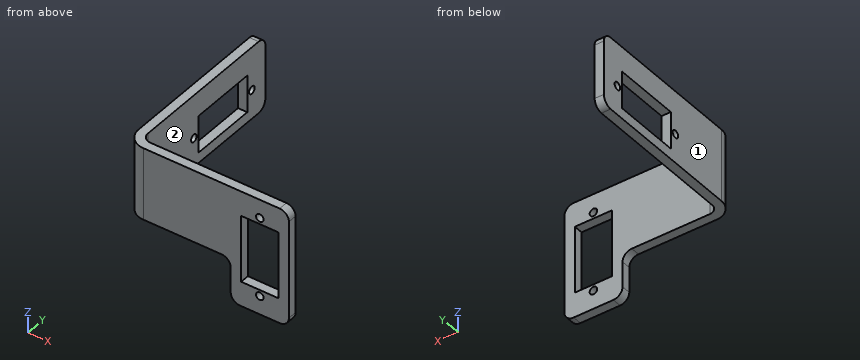
Autodesk Inventor part; units mm, degrees
ref_plane "YZ Plane" through (0, 0, 0) normal (1, 0, 0) x (0, 1, 0)
ref_plane "XZ Plane" through (0, 0, 0) normal (0, 1, 0) x (-1, 0, 0)
ref_plane "XY Plane" through (0, 0, 0) normal (0, 0, 1) x (1, 0, 0)
sketch "Sketch2" plane through (0, 0, 0) normal (0, 1, 0) x (-1, 0, 0)
  line L0 (-6.4, 11.5) -> (6.4, 11.5)
  line L1 (6.4, 11.5) -> (6.4, -11.5)
  line L2 (6.4, -11.5) -> (-6.4, -11.5)
  line L3 (-6.4, -11.5) -> (-6.4, 11.5)
  line L4 (-6.4, 11.5) -> (6.4, -11.5) construction
  line L5 (6.4, 11.5) -> (-6.4, -11.5) construction
  circle A0 centre (0, 0) radius 13.65 construction
  line L6 (0, 0) -> (0, -13.65) construction
  circle A1 centre (0, -13.65) radius 1.3
  circle A2 centre (0, 13.65) radius 1.3
  line L7 (-10, 20) -> (10, 20)
  line L8 (10, 20) -> (10, -20)
  line L9 (10, -20) -> (-10, -20)
  line L10 (-10, -20) -> (-10, 20)
  line L11 (-10, 20) -> (10, -20) construction
  line L12 (10, 20) -> (-10, -20) construction
  line L13 (-10, 5.05) -> (10, 5.05) construction
  line L14 (10, 15.05) -> (100, 15.05)
  line L15 (100, 15.05) -> (100, -4.95)
  line L16 (100, -4.95) -> (10, -4.95)
  line L17 (10, -4.95) -> (10, 15.05)
  line L18 (100, 5.05) -> (10, 5.05) construction
  line L19 (91.5, 11.45) -> (68.5, 11.45)
  line L20 (68.5, 11.45) -> (68.5, -1.35)
  line L21 (68.5, -1.35) -> (91.5, -1.35)
  line L22 (91.5, -1.35) -> (91.5, 11.45)
  line L23 (91.5, 11.45) -> (68.5, -1.35) construction
  line L24 (68.5, 11.45) -> (91.5, -1.35) construction
  circle A3 centre (80, 5.05) radius 13.65 construction
  circle A4 centre (93.65, 5.05) radius 1.3
  circle A5 centre (66.35, 5.05) radius 1.3
  line L25 (100, 15.05) -> (10, 15.05)
  line L26 (10, 15.05) -> (10, 20)
  line L27 (10, 20) -> (100, 20)
  line L28 (100, 20) -> (100, 15.05)
  dimension "d2" = 27.3
  dimension "d20" = 27.3
  dimension "d0" = 12.8
  dimension "d1" = 23
  dimension "d3" = 2.6
  dimension "d6" = 360
  dimension "d8" = 20
  dimension "d9" = 40
  dimension "d11" = 8.6
  dimension "d12" = 90
  dimension "d14" = 20
  dimension "d18" = 12.8
  dimension "d19" = 23
  dimension "d21" = 2.6
  dimension "d24" = 360
  dimension "d26" = 20
extrude "Extrusion1" add sketch "Sketch2" along normal blind 3.175
fillet "Fillet1" radius 3.175 6 edges at (10, 1.5875, 20) (10, 1.5875, -20) (-10, 1.5875, -20) (-10, 1.5875, -4.95) (-100, 1.5875, -4.95) (-100, 1.5875, 20)
sketch "Sketch3" plane through (0, 3.175, 0) normal (0, 1, 0) x (1, 0, 0)
  line L0 (-96.825, -15.05) -> (-13.175, -15.05)
  line L1 (-40, -15.05) -> (-40, 4.95)
  line L2 (-13.175, 4.95) -> (-96.825, 4.95)
  line L3 (10, -16.825) -> (10, 16.825)
  point P0 (0, 0)
  dimension "d27" = 50
bend part "Bend Part1" radius 3 angle 90 line through (-40, 3.175, 15.05) along (0, 0, -1) centre toward (0, 1, 0) moving side (-1, 0, 0) both sides no
equation "\"d20\" = d2"
equation "\"d18\" = d0"
equation "\"d19\" = d1"
equation "\"d21\" = d3"
properties part number "Midplate"
Model file for the job. Use its own axes, mm. Face numbers are marked on the shaded views. A direction names the side the tool comes from. Coordinates: 2 decimals unless noted, no trailing zeros. Order: outer loops, then holes, each group sorted by start corner. A loop starts at its lowest first (then second) coordinate and runs counter-clockwise, first axis right, second up. Notation, with made-up numbers: (51, 0.5) - (59, 0.5) arc R36 ccw to (59, 37.5) - close; hole circle Ø8 at (66, 38.25). An arc over 180 degrees is marked (long way). Return JSON: item names as keys, results as strings. Group by question number.
1) Probe line 1 (Z direction, x = 0, y = 1.85); line 2 (Y direction, x = -44, z = 5); line 3 (Y direction, x = -11, z = 12) (3 decimals). List the from-to ranges inside material, lowest first. Write a range as from..to.
2) Saw through at C-C, the plane z = 5.05. Write the cut outline in (x, y) (3 decimals), plus the area to 3 significant figures.
3) Saw through at D-D, the plane y = 55.5. Write the cut outline in (x, z) (3 decimals), plus the area to 3 significant figures.
4) Saw through at B-B, the plane x = 0.5. Write the cut outline in (y, z) (3 decimals), plus the area to 3 significant figures.
5) Tool access for the marked faces 1 and 2: list every direction of +Z, -Z, +X, -X, +Y, -Y with a clear straight run to the whole face (end or side of a thin tool).
6) Flat gauge pins, fed straight in: P1, Ø6, axis at x = -2.5, z = 5.5, coming from the +Y side; P2, Ø4, axis at x = 0, z = 13.65, coming from the +Y side (3 decimals); P3, Ø1.6, axis at x = -44, y = 47, coming from the -Z side; P4, Ø3, axis at x = 3, z = 11.5, coming from the -Y side. Where does each tip first touch, or does it go through?
7) Saw through at A-A, the plane z = -13.65. Write the cut outline in (x, y) (3 decimals), plus the area to 3 significant figures.
Values found:
{
 "1": {"line 1": "z = -20..-14.95, -12.35..-11.5, 11.5..12.35, 14.95..20", "line 2": "y = 1.47..26.51, 29.11..29.96, 52.96..53.81, 56.41..61.46", "line 3": "y = 0..3.175"},
 "2": {"outline": "(-46.175, 6.175) arc R6.175 ccw to (-40, 0) - (-6.4, 0) - (-6.4, 3.175) - (-40, 3.175) arc R3 cw to (-43, 6.175) - (-43, 26.513) - (-46.175, 26.513) - close; (-46.175, 29.113) - (-43, 29.113) - (-43, 29.963) - (-46.175, 29.963) - close; (-46.175, 52.963) - (-43, 52.963) - (-43, 53.813) - (-46.175, 53.813) - close; (-46.175, 56.413) - (-43, 56.413) - (-43, 61.463) - (-46.175, 61.463) - close; (6.4, 0) - (10, 0) - (10, 3.175) - (6.4, 3.175) - close", "area": "227 mm²"},
 "3": {"outline": "(-46.175, -4.95) - (-43, -4.95) - (-43, 3.809) - (-46.175, 3.809) - close; (-46.175, 6.291) - (-43, 6.291) - (-43, 20) - (-46.175, 20) - close", "area": "71.3 mm²"},
 "4": {"outline": "(0, -20) - (3.175, -20) - (3.175, -14.85) - (0, -14.85) - close; (0, -12.45) - (3.175, -12.45) - (3.175, -11.5) - (0, -11.5) - close; (0, 11.5) - (3.175, 11.5) - (3.175, 12.45) - (0, 12.45) - close; (0, 14.85) - (3.175, 14.85) - (3.175, 20) - (0, 20) - close", "area": "38.7 mm²"},
 "5": {"face 1": "+Z, -Z, -X, +Y, -Y", "face 2": "+Z, -Z, +X, +Y"},
 "6": {"P1": "passes through", "P2": "stops at y = 3.175", "P3": "stops at z = -4.95", "P4": "stops at y = 0"},
 "7": {"outline": "(-10, 0) - (-1.3, 0) - (-1.3, 3.175) - (-10, 3.175) - close; (1.3, 0) - (10, 0) - (10, 3.175) - (1.3, 3.175) - close", "area": "55.2 mm²"}
}
